The model under review builds one solid part; all positions refer to its coordinate system, in mm. A direction names the side the tool comes from. Give positions to 0.01 mm unless a question says otherwise; leave off trailing zeros. Order: outer loops, then holes, each group sorted by start corner. A loop starts at its lowest first (then second) coordinate and runs counter-clockwise, first axis right, second up. Notation, with made-up numbers: (6.5, -19.5) -> (36.5, -19.5) arc R19 cw to (36.5, 14.5) -> close; hole circle Ø1 at (-18.5, 6.5). An arc over 180 degrees is marked (long way). Answer as a JSON object with one key per item and string values. Group by question number.
from build123d import *

# Parameters (mm, degrees)
SKETCH1_W           = 67.31
SKETCH1_H           = 41.91
BOSS_EXTRUDE5_DEPTH = 3.175
SKETCH2_W           = 67.31
SKETCH2_H           = 41.91
SKETCH2_W_2         = 60.96
SKETCH2_H_2         = 35.56
BOSS_EXTRUDE6_DEPTH = 7.62
SKETCH4_W           = 12.7
SKETCH4_H           = 6.35
SKETCH4_W_2         = 6.35
SKETCH4_H_2         = 12.7
BOSS_EXTRUDE8_DEPTH = 3.175
SKETCH6_R           = 1.5875
CUT_EXTRUDE1_DEPTH  = 50.62353348
SKETCH7_W           = 3
SKETCH7_H           = 3
CUT_EXTRUDE2_DEPTH  = 77.355944595


with BuildPart() as part:
    # Sketch1 → Boss-Extrude5 (new body)
    with BuildSketch(Plane(origin=(0, 0, 0), x_dir=(1, 0, 0), z_dir=(0, 1, 0))):
        Rectangle(SKETCH1_W, SKETCH1_H)
    extrude(amount=BOSS_EXTRUDE5_DEPTH)

    # Sketch2 → Boss-Extrude6 (add)
    with BuildSketch(Plane(origin=(0, 3.175, 0), x_dir=(1, 0, 0), z_dir=(0, 1, 0))):
        Rectangle(SKETCH2_W, SKETCH2_H)
        Rectangle(SKETCH2_W_2, SKETCH2_H_2, mode=Mode.SUBTRACT)
    extrude(amount=BOSS_EXTRUDE6_DEPTH)

    # Sketch4 → Boss-Extrude8 (add)
    with BuildSketch(Plane(origin=(0, 10.795, 0), x_dir=(1, 0, 0), z_dir=(0, 1, 0))):
        with Locations((0, -24.13)):
            Rectangle(SKETCH4_W, SKETCH4_H)
        with Locations((0, 24.13)):
            Rectangle(SKETCH4_W, SKETCH4_H)
        with Locations((36.83, 0)):
            Rectangle(SKETCH4_W_2, SKETCH4_H_2)
        with Locations((-36.83, 0)):
            Rectangle(SKETCH4_W_2, SKETCH4_H_2)
    extrude(amount=-BOSS_EXTRUDE8_DEPTH)

    # Sketch6 → Cut-Extrude1 (cut, through all)
    with BuildSketch(Plane(origin=(0, 10.795, 0), x_dir=(1, 0, 0), z_dir=(0, 1, 0))):
        with BuildLine():
            ThreePointArc((0, 25.7175), (-1.5875, 24.13), (0, 22.5425))
            Line((0, 22.5425), (0, 25.7175))
        make_face()
        with BuildLine():
            Line((0, 25.7175), (0, 22.5425))
            ThreePointArc((0, 22.5425), (1.122532015, 23.007467985), (1.5875, 24.13))
            ThreePointArc((1.5875, 24.13), (1.122532015, 25.252532015), (0, 25.7175))
        make_face()
        with Locations(Location((-36.806414665, 0, 0), (0, 0, 270))):
            Circle(SKETCH6_R)
        with Locations(Location((36.83, 0, 0), (0, 0, 270))):
            Circle(SKETCH6_R)
        with Locations(Location((0, -24.13, 0), (0, 0, 270))):
            Circle(SKETCH6_R)
    extrude(amount=-CUT_EXTRUDE1_DEPTH, mode=Mode.SUBTRACT)

    # Sketch7 → Cut-Extrude2 (cut, through all)
    with BuildSketch(Plane(origin=(-30.48, 0, 0), x_dir=(0, 0, -1), z_dir=(1, 0, 0))):
        with Locations((12.065620766, 6.985)):
            Rectangle(SKETCH7_W, SKETCH7_H)
    extrude(amount=-CUT_EXTRUDE2_DEPTH, mode=Mode.SUBTRACT)


solid = part.part
1. Machinability: for faces 1 (the flat face through (-38, 7.62, -2)), 2 (the flat face through (-6.35, 9, 24)), 3 (the flat face through (-2, 7.62, -25)), 4 (the flat face through (37, 9, 6.35)), 5 (the flat face through (0, 3.175, 0)), which of the approach directions +Z, -Z, +X, -X, +Y, -Y give a long, thin tool a straight path to every point of the face, cutting with its end or side? Answer none if there is none.
2. For probe 1 along X at (y, z) = (9.2, 0) (1 decimal); probe 2 along X at (y, z) = (6.25, -15) (3 decimals); probe 3 along Z at (x, y) = (-25, 3.75) (3 decimals), list the stretches that pass through material, from the lowest coordinate up. Write a range as [from, to].
3. Take a section at D-D on z = 16. Give the boundary of the cut face in (x, y) (3 decimals).
4. For pin 1 (1 mm diameter, centred on x = -37, y = 8.5, fed in from +Z); pin 2 (1.5 mm diameter, centred on x = -31.5, y = 7, fed in from -Z) (3 decimals); pin 3 (10 mm diameter, centred on x = -19.5, z = -3, fed in from +Y) (3 decimals), all flat-tipped, find the tip position at first contact; note any pin that passes through.
5. Draft analysis for pull direction X (two halves, no side actions). For faces 6 (the flat face through (-6.35, 9, -24)), 7 (the flat face through (-32, 5.485, -12)), 8 (the flat face through (30.48, 7, 0)), state which applies: pulls with the +X half, pulls with the -X half, needs draft (parallel to the pull), parting line crosses it, or undercut.
6. Take a section at C-C on y = 4.5. Give the boundary of the cut face in (x, z) (3 decimals), plus the area to 3 significant figures.
Checks:
{
 "1": {"face 1": "+Z, -Z, -X, -Y", "face 2": "+Z, -X, +Y, -Y", "face 3": "-Z, +X, -X, -Y", "face 4": "+Z, +X, +Y, -Y", "face 5": "+Y"},
 "2": {"probe 1": "x = [-40, -38.4], [-35.2, -30.5], [30.5, 35.2], [38.4, 40]", "probe 2": "x = [-33.655, -30.48], [30.48, 33.655]", "probe 3": "z = [-20.955, -17.78], [17.78, 20.955]"},
 "3": {"outline": "(-33.655, 0) -> (33.655, 0) -> (33.655, 10.795) -> (30.48, 10.795) -> (30.48, 3.175) -> (-30.48, 3.175) -> (-30.48, 10.795) -> (-33.655, 10.795) -> close"},
 "4": {"pin 1": "stops at z = 6.35", "pin 2": "stops at z = -20.955", "pin 3": "stops at y = 3.175"},
 "5": {"face 6": "pulls with the -X half", "face 7": "needs draft", "face 8": "undercut"},
 "6": {"outline": "(-33.655, -20.955) -> (33.655, -20.955) -> (33.655, 20.955) -> (-33.655, 20.955) -> close; hole (-30.48, -17.78) -> (30.48, -17.78) -> (30.48, 17.78) -> (-30.48, 17.78) -> close", "area": "653 mm2"}
}
